from build123d import *

# Parameters (mm, degrees)
SKETCH1_W           = 71
SKETCH1_H           = 63
SKETCH1_R           = 2.1
SKETCH1_W_2         = 20.991665644
SKETCH1_H_2         = 40.2
SKETCH1_W_3         = 21
BOSS_EXTRUDE1_DEPTH = 4


with BuildPart() as part:
    # Sketch1 → Boss-Extrude1 (new body)
    with BuildSketch(Plane(origin=(0, 0, 0), x_dir=(1, 0, 0), z_dir=(0, 1, 0))):
        with Locations((-62.085116344, -11.139897002)):
            Rectangle(SKETCH1_W, SKETCH1_H)
        with Locations((-80.035116344, 12.860102998)):
            Circle(SKETCH1_R, mode=Mode.SUBTRACT)
        with Locations((-70.135116344, 12.860102998)):
            Circle(SKETCH1_R, mode=Mode.SUBTRACT)
        with Locations((-54.035116344, 12.860102998)):
            Circle(SKETCH1_R, mode=Mode.SUBTRACT)
        with Locations((-44.135116344, 12.860102998)):
            Circle(SKETCH1_R, mode=Mode.SUBTRACT)
        with Locations((-30.585116344, 4.860102998)):
            Circle(SKETCH1_R, mode=Mode.SUBTRACT)
        with Locations((-93.585116344, 4.860102998)):
            Circle(SKETCH1_R, mode=Mode.SUBTRACT)
        with Locations((-30.585116344, -27.139897002)):
            Circle(SKETCH1_R, mode=Mode.SUBTRACT)
        with Locations((-44.135116344, -35.139897002)):
            Circle(SKETCH1_R, mode=Mode.SUBTRACT)
        with Locations((-54.035116344, -35.139897002)):
            Circle(SKETCH1_R, mode=Mode.SUBTRACT)
        with Locations((-80.035116344, -35.139897002)):
            Circle(SKETCH1_R, mode=Mode.SUBTRACT)
        with Locations((-70.135116344, -35.139897002)):
            Circle(SKETCH1_R, mode=Mode.SUBTRACT)
        with Locations((-93.585116344, -27.139897002)):
            Circle(SKETCH1_R, mode=Mode.SUBTRACT)
        with Locations((-75.080949166, -11.139897002)):
            Rectangle(SKETCH1_W_2, SKETCH1_H_2, mode=Mode.SUBTRACT)
        with Locations((-49.085116344, -11.139897002)):
            Rectangle(SKETCH1_W_3, SKETCH1_H_2, mode=Mode.SUBTRACT)
    extrude(amount=BOSS_EXTRUDE1_DEPTH)


solid = part.part
The listing builds one solid part. Answer for the finished solid, in the listing's coordinates (mm). A direction names the side the tool comes from. Coordinates: 2 decimals unless noted, no trailing zeros. Loops run counter-clockwise (first coordinate to the right, second up) from the corner with the lowest first, then second, coordinate; pieces in that order, holes last. Notation, with made-up numbers: (71.5, 61) -> (83.5, 61) arc R7 cw to (83.5, 65) -> close; hole circle Ø4 at (-33, -33.5). An arc over 180 degrees is marked (long way). Answer in a Markdown table with one row per item. Add a question column.
1. Consider line 1 (X direction, y = 0.95, z = 25); line 2 (Z direction, x = -70, y = 0.8); line 3 (Z direction, x = -46, y = 0.2). Determine where each line is inside the solid, lowest interval first. Write a range as [from, to].
2. Determine the mould class of faces 3 (the flat face through (-26.585, 2, 12)), 4 (the flat face through (-63, 0, 11)), 5 (the cylindrical face through (-71.8, 1.97, 36.42)) for opening direction X: +X half, -X half, draft (parallel to the pull), parting line (faces both ways), or undercut.
3. The part is cut by section C-C, the plane y = 1.25. Count the separate pieces of the cut face and the enclosed holes in it, then the cut area to 3 significant figures.
4. The part is cut by section B-B, the plane x = -45. Write down the section's boundary in (y, z).
5. For faces 1 (the flat face through (-38.585, 2, 11)), 2 (the flat face through (-63, 2, -20.36)), determine the directions among +Z, -Z, +X, -X, +Y, -Y from which every point of the face is accessible in a straight line to the end or side of a thin tool.
6. The part is cut by section A-A, the plane z = 3.5. Write down the section's boundary in (x, y), then the cut area to 3 significant figures.
7. A flat-ended cylindrical pin translates along its axis: P1, Ø4, axis at x = -70.14, z = -12.86, coming from the +Y side. Find the tip coordinate at first contact, or state that the pin passes through.
Answer below:
| question | item | result |
|---|---|---|
| 1 | line 1 | [-97.59, -85.58], [-64.59, -59.59], [-38.59, -26.59] |
| 1 | line 2 | [-20.36, -14.96], [-10.76, -8.96], [31.24, 33.04], [37.24, 42.64] |
| 1 | line 3 | [-20.36, -13.83], [-11.89, -8.96], [31.24, 34.17], [36.11, 42.64] |
| 2 | face 3 | +X half |
| 2 | face 4 | draft |
| 2 | face 5 | undercut |
| 3 | separate pieces | 1 |
| 3 | enclosed holes | 14 |
| 3 | area | 2,620 mm2 |
| 4 | outline | (0, -20.36) -> (4, -20.36) -> (4, -14.77) -> (0, -14.77) -> close; (0, -10.95) -> (4, -10.95) -> (4, -8.96) -> (0, -8.96) -> close; (0, 31.24) -> (4, 31.24) -> (4, 33.23) -> (0, 33.23) -> close; (0, 37.05) -> (4, 37.05) -> (4, 42.64) -> (0, 42.64) -> close |
| 5 | face 1 | +Y, -Y |
| 5 | face 2 | -Z, +X, -X, +Y, -Y |
| 6 | outline | (-97.59, 0) -> (-85.58, 0) -> (-85.58, 4) -> (-97.59, 4) -> close; (-64.59, 0) -> (-59.59, 0) -> (-59.59, 4) -> (-64.59, 4) -> close; (-38.59, 0) -> (-26.59, 0) -> (-26.59, 4) -> (-38.59, 4) -> close |
| 6 | area | 116 mm2 |
| 7 | P1 | through |
